```python
from build123d import *

# Parameters (mm, degrees)
SKETCH1_R                = 7.62
BOSS_EXTRUDE1_DEPTH      = 10.16
SKETCH3_R                = 8.7376
SKETCH3_R_2              = 3.27025
BOSS_EXTRUDE2_DEPTH      = 1.5875
BOSS_EXTRUDE2_DEPTH_BACK = 1.5875
SKETCH4_R                = 1.98374
CUT_EXTRUDE1_DEPTH       = 10.16


with BuildPart() as part:
    # Sketch1 → Boss-Extrude1 (new body)
    with BuildSketch(Plane.XY):
        with BuildLine():
            Line((0, 0), (-18.923, 0))
            Line((-18.923, 0), (-18.923, 8.382))
            Line((-18.923, 8.382), (-11.43, 15.875))
            ThreePointArc((-11.43, 15.875), (0, 27.305), (11.43, 15.875))
            Line((11.43, 15.875), (18.923, 8.382))
            Line((18.923, 8.382), (18.923, 0))
            Line((18.923, 0), (0, 0))
        make_face()
        with Locations((0, 15.875)):
            Circle(SKETCH1_R, mode=Mode.SUBTRACT)
    extrude(amount=BOSS_EXTRUDE1_DEPTH)

    # Sketch3 → Boss-Extrude2 (add, two sides)
    with BuildSketch(Plane.XY.offset(5.08)) as boss_extrude2_sk:
        with Locations((0, 15.875)):
            Circle(SKETCH3_R)
        with Locations((0, 15.875)):
            Circle(SKETCH3_R_2, mode=Mode.SUBTRACT)
    extrude(amount=BOSS_EXTRUDE2_DEPTH)
    extrude(boss_extrude2_sk.sketch, amount=-BOSS_EXTRUDE2_DEPTH_BACK)

    # Sketch4 → Cut-Extrude1 (cut)
    with BuildSketch(Plane(origin=(0, 0, 0), x_dir=(-1, 0, 0), z_dir=(0, -1, 0))):
        with Locations((-10.16, -5.08)):
            Circle(SKETCH4_R)
        with Locations((10.16, -5.08)):
            Circle(SKETCH4_R)
    extrude(amount=-CUT_EXTRUDE1_DEPTH, mode=Mode.SUBTRACT)


solid = part.part
```
Design review of the part built by this model. Coordinates are the model's own, in mm. A direction names the side the tool comes from. Give positions to 0.01 mm unless a question says otherwise; leave off trailing zeros. Order: outer loops, then holes, each group sorted by start corner. A loop starts at its lowest first (then second) coordinate and runs counter-clockwise, first axis right, second up. Notation, with made-up numbers: (56, -25.75) -> (106, -25.75) arc R10 cw to (106, -14.75) -> close; hole circle Ø9 at (77.25, -36.75). An arc over 180 degrees is marked (long way). Write each question's results on one line, items separated by ' | '. Start each with the question number.
Q1. Add section D-D on x = -4.5. Give the boundary of the cut face in (y, z), and give its area (3 significant figures).
Q2. Machinability: for faces 4 (the flat face through (3, 14, 6.668)), 5 (the cylindrical face through (-11.075, 5.009, 6.84)), 6 (the flat face through (18.923, 4, 5)), 7 (the cylindrical face through (-0.99, 23.43, 1.72)), which of the approach directions +Z, -Z, +X, -X, +Y, -Y give a long, thin tool a straight path to every point of the face, cutting with its end or side? Answer none if there is none.
Q3. Mouldability with a two-part tool opening along X and no side actions: class faces 1 (the flat face through (-18.923, 4, 5)), 2 (the flat face through (0, 8, 10.16)), 3 (the flat face through (-10, 10.16, 5)) as +X half, -X half, draft (parallel to the pull), parting line (faces both ways), or undercut.
Q4. Add section A-A on x = 0. Give the boundary of the cut face in (y, z) (1 decimal).
Q5. Wall thickness on L1, parallel to X at y = 2.75, z = 5.08; L2, parallel to X at y = 16.25, z = 8.25; L3, parallel to Y at x = 0, z = 0.8 (3 decimals): over which ranges is each line inside the solid? List them lowest first. Write a range as from..to.
Q6. Add section B-B on z = 1.5. Give the boundary of the cut face in (x, y) (3 decimals).
Q7. Add section C-C on y = 2.5. Give the boundary of the cut face in (x, z).
Q8. For pin 1 (1 mm diameter, centred on y = 10, z = 8.5, fed in from -X) (3 decimals); pin 2 (13.5 mm diameter, centred on x = 0, y = 15.875, fed in from +Z); pin 3 (1.5 mm diameter, centred on y = 16.5, z = 7.5, fed in from +X) (3 decimals), all flat-tipped, find the tip position at first contact; note any pin that passes through.
Found:
1) outline: (0, 0) -> (9.73, 0) -> (9.73, 3.49) -> (22.02, 3.49) -> (22.02, 0) -> (26.38, 0) -> (26.38, 10.16) -> (22.02, 10.16) -> (22.02, 6.67) -> (9.73, 6.67) -> (9.73, 10.16) -> (0, 10.16) -> close | area: 182 mm2
2) face 4: +Z | face 5: -Y | face 6: +Z, -Z, +X, +Y, -Y | face 7: -Z
3) face 1: -X half | face 2: draft | face 3: undercut
4) outline: (0, 0) -> (8.3, 0) -> (8.3, 3.5) -> (12.6, 3.5) -> (12.6, 6.7) -> (8.3, 6.7) -> (8.3, 10.2) -> (0, 10.2) -> close; (19.1, 3.5) -> (23.5, 3.5) -> (23.5, 0) -> (27.3, 0) -> (27.3, 10.2) -> (23.5, 10.2) -> (23.5, 6.7) -> (19.1, 6.7) -> close
5) L1: x = -18.92..-12.14, -8.18..8.18, 12.14..18.92 | L2: x = -11.42..-7.61, 7.61..11.42 | L3: y = 0..8.255, 23.495..27.305
6) outline: (-18.923, 0) -> (18.923, 0) -> (18.923, 8.382) -> (11.43, 15.875) arc R11.43 ccw to (-11.43, 15.875) -> (-18.923, 8.382) -> close; hole circle Ø15.24 at (0, 15.875)
7) outline: (-18.92, 0) -> (18.92, 0) -> (18.92, 10.16) -> (-18.92, 10.16) -> close; hole circle Ø3.97 at (-10.16, 5.08); hole circle Ø3.97 at (10.16, 5.08)
8) pin 1: stops at x = -17.805 | pin 2: stops at z = 6.67 | pin 3: stops at x = 11.555
